The listing builds one solid part. Answer for the finished solid, in the listing's coordinates (mm). Face numbers are marked on the shaded views. Coordinates: 2 decimals unless noted, no trailing zeros. Loops run counter-clockwise (first coordinate to the right, second up) from the corner with the lowest first, then second, coordinate; pieces in that order, holes last. Notation, with made-up numbers: (73.25, 46) - (86.25, 46) arc R13 ccw to (86.25, 70) - close; hole circle Ø7 at (-16.5, -18). An arc over 180 degrees is marked (long way). Return JSON: item names as keys, results as strings. Group by question number.
1. Section A-A (z = 8.25) is taken. Write down the section's boundary in (x, y).
2. Each of these flat-tipped pins is pushed along its axis until it touches: P1, Ø1, axis at y = 10.5, z = 8.5, coming from the -X side; P2, Ø0.5, axis at y = -8, z = 5.5, coming from the +X side; P3, Ø5, axis at x = 34.5, y = 0.5, coming from the +Z side; P4, Ø10, axis at x = -19, y = -3, coming from the -Z side. Where does it stop, or does it pass through?
3. The mould has two halves that part along Z. Classify the marked faces 1, 2 and 3: pulls with the +Z half, pulls with the -Z half, needs draft (parallel to the pull), parting line crosses it, or undercut.
4. Find the intervals of material crossed by line 1 along Y through (x, z) = (34.5, 5.5); line 2 along X through (y, z) = (-3, 8.5), in increasing order.
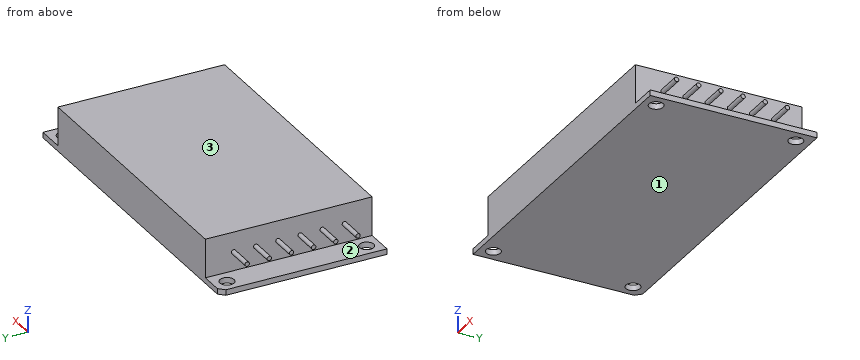
```python
from build123d import *

# Parameters (mm, degrees)
F0_W      = 76.327
F0_H      = 38.227
F1_DEPTH  = 1.27
F2_W      = 63.5
F2_H      = 38.227
F3_DEPTH  = 8.89
F5_D      = 3.2512
F6_D      = 3.2512
F8_D      = 3.2512
F9_D      = 3.2512
F10_R     = 0.508
F12_DEPTH = 5.842
F11_R     = 0.508
F13_DEPTH = 5.842
F14_SIZE  = 1.27


with BuildPart() as f1:
    # F0 (on Top) → F1 (new body)
    with BuildSketch(Plane.XY):
        Rectangle(F0_W, F0_H)
    extrude(amount=F1_DEPTH)

    # F2 (on face) → F3 (join)
    with BuildSketch(Plane.XY.offset(1.27)):
        Rectangle(F2_W, F2_H)
    extrude(amount=F3_DEPTH)

    # F5 (through all)
    with Locations(Plane.XY.offset(1.27)):
        with Locations((34.9885, -16.0655)):
            Hole(F5_D / 2)

    # F6 (through all)
    with Locations(Plane.XY.offset(1.27)):
        with Locations((34.9885, 15.9385)):
            Hole(F6_D / 2)

    # F8 (through all)
    with Locations(Plane.XY.offset(1.27)):
        with Locations((-35.1155, -16.0655)):
            Hole(F8_D / 2)

    # F9 (through all)
    with Locations(Plane.XY.offset(1.27)):
        with Locations((-35.1155, 15.9385)):
            Hole(F9_D / 2)

    # F10 (on face) → F12 (join)
    with BuildSketch(Plane.YZ.offset(31.75)):
        with Locations((-12.7635, 5.588)):
            Circle(F10_R)
        with Locations((-7.6835, 5.588)):
            Circle(F10_R)
        with Locations((-2.6035, 5.588)):
            Circle(F10_R)
        with Locations((2.4765, 5.588)):
            Circle(F10_R)
        with Locations((7.5565, 5.588)):
            Circle(F10_R)
        with Locations((12.6365, 5.588)):
            Circle(F10_R)
    extrude(amount=F12_DEPTH)

    # F11 (on face) → F13 (join)
    with BuildSketch(Plane(origin=(-31.75, 0, 0), x_dir=(0, -1, 0), z_dir=(-1, 0, 0))):
        with Locations((-12.6365, 5.588)):
            Circle(F11_R)
        with Locations((-7.5565, 5.588)):
            Circle(F11_R)
        with Locations((-2.4765, 5.588)):
            Circle(F11_R)
        with Locations((2.6035, 5.588)):
            Circle(F11_R)
        with Locations((7.6835, 5.588)):
            Circle(F11_R)
        with Locations((12.7635, 5.588)):
            Circle(F11_R)
    extrude(amount=F13_DEPTH)

    # F14
    f14_edges = [f1.edges().sort_by_distance(p)[0] for p in [
        (-38.1635, 19.1135, 0.635),
    ]]
    chamfer(f14_edges, length=F14_SIZE)


solid = f1.part
```
The answers:
{
 "1": {"outline": "(-31.75, -19.11) - (31.75, -19.11) - (31.75, 19.11) - (-31.75, 19.11) - close"},
 "2": {"P1": "stops at x = -31.75", "P2": "stops at x = 37.59", "P3": "stops at z = 6.1", "P4": "stops at z = 0"},
 "3": {"face 1": "pulls with the -Z half", "face 2": "undercut", "face 3": "pulls with the +Z half"},
 "4": {"line 1": "y = -13.26 to -12.26, -8.18 to -7.18, -3.1 to -2.1, 1.98 to 2.98, 7.06 to 8.06, 12.14 to 13.14", "line 2": "x = -31.75 to 31.75"}
}
